Input: dimensioned drawing with shaded views. Units: mm. Origin: part minimum x, y, z. Coordinates: 2 decimals unless noted, no trailing zeros. Loops run counter-clockwise (first coordinate to the right, second up) from the corner with the lowest first, then second, coordinate; pieces in that order, holes last. Notation, with made-up numbers: (86.5, -4.75) - (109.5, -4.75) arc R20 cw to (109.5, 13.25) - close; hole circle Ø11 at (70.5, -25). An arc over 180 degrees is marked (long way). Put each result on its own line as item: value. Start each with the question number.
1) Draft query along Y for the marked faces 1, 2 and 3. Return one class per face: +Y half, -Y half, draft (parallel to the pull), parting line (faces both ways), or undercut.
2) Material intervals for line 1 along X through (y, z) = (0.5, 8); line 2 along X through (y, z) = (1.15, 15.5); line 3 along Y through (x, z) = (11.5, 20.75), sorted ascending. Write a range as from..to.
3) Section D-D on y = 0.6. Output: boundary loops of the cut face in (x, z).
4) Section C-C on z = 19. Output: boundary loops of the cut face in (x, y).
5) Contact query for flat-ended pins moving along their axis: pin 1 Ø1.2 at (y, z) = (0.5, 8) entering from -X; pin 2 Ø1.5 at (y, z) = (3, 20) entering from +X; pin 3 Ø2 at (x, z) = (8, 14) entering from -Y. Output: stop coordinate, or through.
6) Section A-A on z = 14.25. Output: boundary loops of the cut face in (x, y).
7) Section B-B on x = 4.25. Output: boundary loops of the cut face in (y, z).
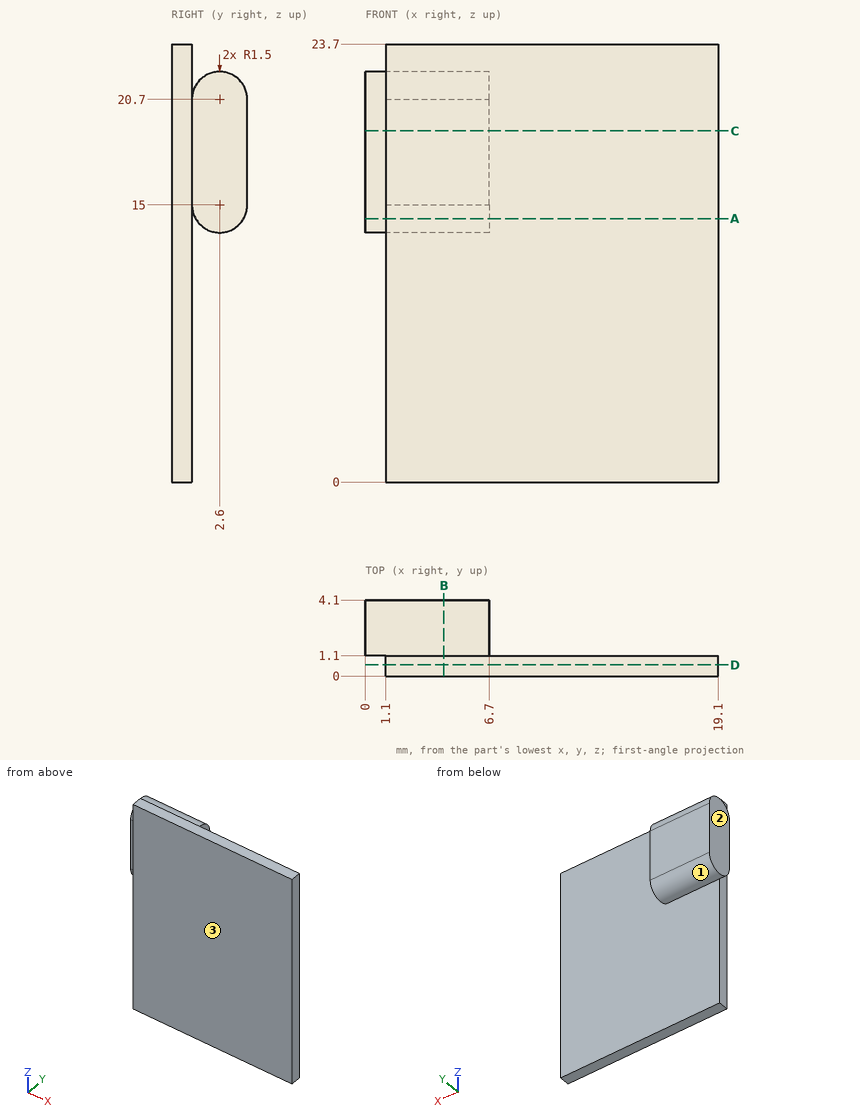
Answer block:
1. face 1: undercut
1. face 2: draft
1. face 3: -Y half
2. line 1: x = 1.1..19.1
2. line 2: x = 0..6.7
2. line 3: y = 0..1.1
3. outline: (1.1, 0) - (19.1, 0) - (19.1, 23.7) - (1.1, 23.7) - close
4. outline: (0, 1.1) - (1.1, 1.1) - (1.1, 0) - (19.1, 0) - (19.1, 1.1) - (6.7, 1.1) - (6.7, 4.1) - (0, 4.1) - close
5. pin 1: stops at x = 1.1
5. pin 2: stops at x = 6.7
5. pin 3: stops at y = 0
6. outline: (0, 1.3) - (6.7, 1.3) - (6.7, 3.9) - (0, 3.9) - close; (1.1, 0) - (19.1, 0) - (19.1, 1.1) - (1.1, 1.1) - close
7. outline: (0, 0) - (1.1, 0) - (1.1, 15) arc R1.5 ccw to (4.1, 15) - (4.1, 20.7) arc R1.5 ccw to (1.1, 20.7) - (1.1, 23.7) - (0, 23.7) - close
